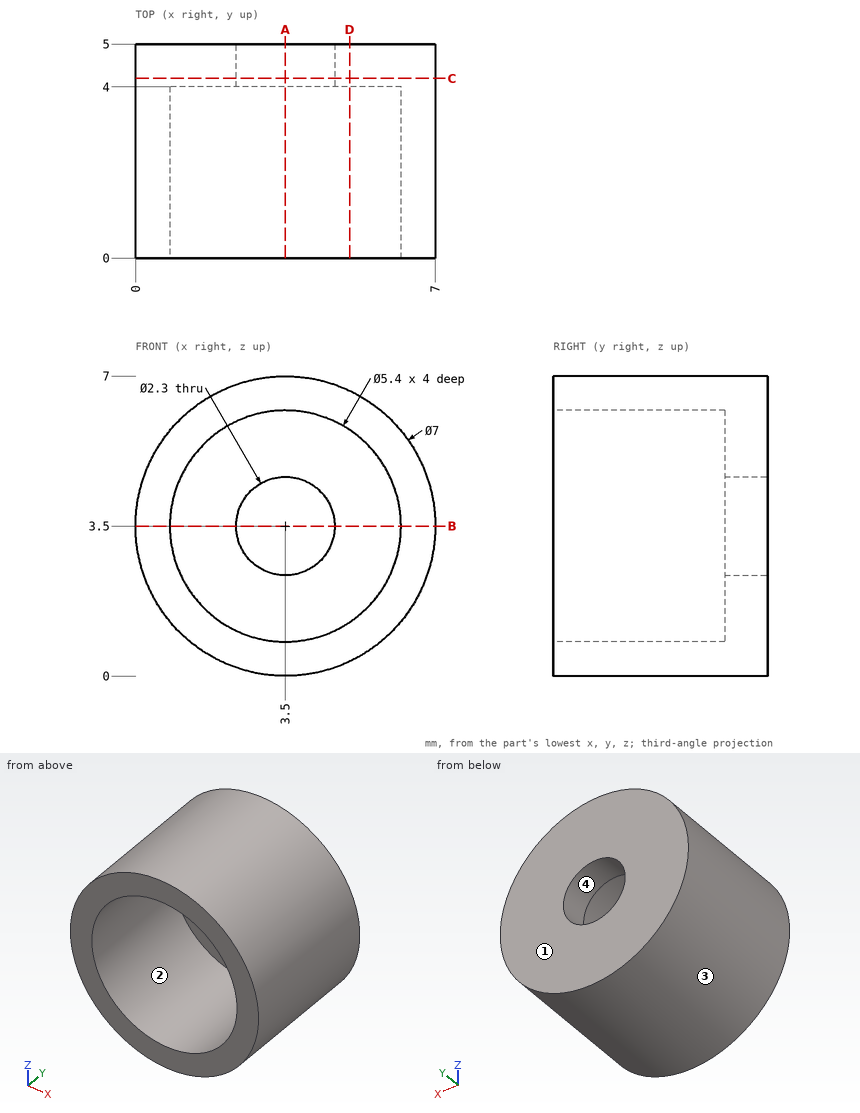
Check sheet for the drawn part. Datum: minimum x, y, z corner. Units: mm. Coordinates: 2 decimals unless noted, no trailing zeros. Order: outer loops, then holes, each group sorted by start corner. A loop starts at its lowest first (then second) coordinate and runs counter-clockwise, first axis right, second up. Notation, with made-up numbers: M 31,-20 L 38,-20 A28 cw 38,11 Z; hole C 51.5,40 d9. An arc over 180 degrees is marked long. One line per question, with ' | ' between items. Start each with the question number.
Item 1: Cross-section at D-D on x = 5. Enter the section's corners in (y, z) (3 decimals).
Item 2: Cross-section at C-C on y = 4.2. Enter the section's corners in (x, z).
Item 3: Cross-section at B-B on z = 3.5. Enter the section's corners in (x, y), then the cut area to 3 significant figures.
Item 4: Draft check along Z on the marked faces 1, 2, 3 and 4. Enter one of: pulls with the +Z half, pulls with the -Z half, needs draft (parallel to the pull), parting line crosses it, or undercut.
Item 5: Cross-section at A-A on x = 3.5. Enter the section's corners in (y, z), then the cut area to 3 significant figures.
Item 6: Material ranges on L1, parallel to Z at x = 3.5, y = 4.6; L2, parallel to Z at x = 3.5, y = 1.5; L3, parallel to Y at x = 2.5, z = 2, recorded low to high. Write a range as [from, to].
Findings:
1) outline: M 0,0.338 L 5,0.338 L 5,6.662 L 0,6.662 L 0,5.745 L 4,5.745 L 4,1.255 L 0,1.255 Z
2) outline: C 3.5,3.5 d7; hole C 3.5,3.5 d2.3
3) outline: M 0,0 L 0.8,0 L 0.8,4 L 2.35,4 L 2.35,5 L 0,5 Z; M 4.65,4 L 6.2,4 L 6.2,0 L 7,0 L 7,5 L 4.65,5 Z | area: 11.1 mm²
4) face 1: needs draft | face 2: undercut | face 3: parting line crosses it | face 4: undercut
5) outline: M 0,0 L 5,0 L 5,2.35 L 4,2.35 L 4,0.8 L 0,0.8 Z; M 0,6.2 L 4,6.2 L 4,4.65 L 5,4.65 L 5,7 L 0,7 Z | area: 11.1 mm²
6) L1: z = [0, 2.35], [4.65, 7] | L2: z = [0, 0.8], [6.2, 7] | L3: y = [4, 5]
